Design review of the part built by this model. Coordinates are the model's own, in mm. Give positions to 0.01 mm unless a question says otherwise; leave off trailing zeros. Write each loop counter-clockwise with the first axis right and the second up, starting at its lowest first coordinate (ties: lowest second). Pieces come first, ordered by that corner, then holes. Notation, with made-up numbers: (52.5, 63.5) - (85.5, 63.5) arc R9 cw to (85.5, 69.5) - close; hole circle Ø7 at (54, 55). An arc over 180 degrees is marked (long way). Write each question's results on one line, items separated by ' | '. Start each with the question number.
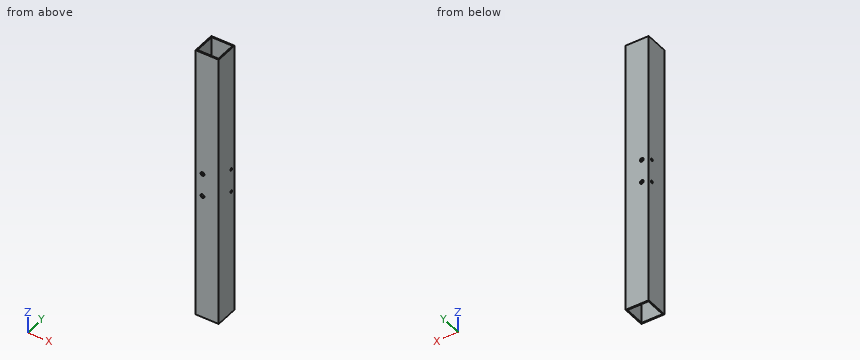
from build123d import *

# Parameters (mm, degrees)
SKETCH1_W               = 20
SKETCH1_H               = 20
SKETCH1_W_2             = 18
SKETCH1_H_2             = 18
BOSS_EXTRUDE2_DEPTH     = 238.73
CUT_EXTRUDE1_DEPTH      = 240.774921332
CUT_EXTRUDE1_DEPTH_BACK = 240.774921332
SKETCH3_R               = 1.65
CUT_EXTRUDE2_DEPTH      = 240.774921332
CUT_EXTRUDE2_DEPTH_BACK = 240.774921332
SKETCH4_R               = 1.15


with BuildPart() as part:
    # Sketch1 → Boss-Extrude2 (new body)
    with BuildSketch(Plane.XY):
        Rectangle(SKETCH1_W, SKETCH1_H)
        Rectangle(SKETCH1_W_2, SKETCH1_H_2, mode=Mode.SUBTRACT)
    extrude(amount=BOSS_EXTRUDE2_DEPTH)

    # Sketch3 → Cut-Extrude1 (cut, two sides: drawn at the far end of the back side and taken through both)
    with BuildSketch(Plane(origin=(0, 10, 0), x_dir=(1, 0, 0), z_dir=(0, 1, 0)).offset(-CUT_EXTRUDE1_DEPTH_BACK)):
        with Locations(Location((-4, -109.46, 0), (0, 0, 270))):
            Circle(SKETCH3_R)
        with Locations(Location((-4, -129.46, 0), (0, 0, 270))):
            Circle(SKETCH3_R)
    extrude(amount=CUT_EXTRUDE1_DEPTH + CUT_EXTRUDE1_DEPTH_BACK, mode=Mode.SUBTRACT)

    # Sketch4 → Cut-Extrude2 (cut, two sides: drawn at the far end of the back side and taken through both)
    with BuildSketch(Plane.ZY.offset(10).offset(-CUT_EXTRUDE2_DEPTH_BACK)):
        with Locations(Location((129.47, 6, 0), (0, 0, 180))):
            Circle(SKETCH4_R)
        with Locations(Location((109.47, 6, 0), (0, 0, 180))):
            Circle(SKETCH4_R)
    extrude(amount=CUT_EXTRUDE2_DEPTH + CUT_EXTRUDE2_DEPTH_BACK, mode=Mode.SUBTRACT)


solid = part.part
Q1. Add section A-A on y = -4. State the section outline as (x, z) points.
Q2. Insertion check: P1, Ø3.5, axis at y = 6, z = 129.47, coming from the +X side. The pin has a flat end and moves straight along its axis. Give the tip position at first contact, or say it passes through.
Q3. Add section C-C on z = 199.5. State the section outline as (x, y) points.
Q4. For line 1 along Z through (x, y) = (-4, -9.35); line 2 along Y through (x, z) = (5.5, 155.5), list the stretches that pass through material, from the lowest coordinate up. Write a range as [from, to].
Result:
1) outline: (-10, 0) - (-9, 0) - (-9, 238.73) - (-10, 238.73) - close; (9, 0) - (10, 0) - (10, 238.73) - (9, 238.73) - close
2) P1: stops at x = 10
3) outline: (-10, -10) - (10, -10) - (10, 10) - (-10, 10) - close; hole (-9, -9) - (9, -9) - (9, 9) - (-9, 9) - close
4) line 1: z = [0, 107.81], [111.11, 127.81], [131.11, 238.73] | line 2: y = [-10, -9], [9, 10]
